```python
from build123d import *

# Parameters (mm, degrees)
F1_DEPTH       = 12.065
F2_R           = 9.525
F3_DEPTH       = 15.25
F4_R           = 9.625
F5_DEPTH       = 25
F7_D           = 9
F7_DEPTH       = 75
F7_CBORE_D     = 11
F7_CBORE_DEPTH = 5
F7_TIP         = 2.7038727856
F8_R           = 2.5


# Not quite as in the source:
# - a pattern or mirror of a feature is missing from the dataset's text; its kind, count and spacing are read off the source's solid


with BuildPart() as f1:
    # F0 (on Right) → F1 (new body, symmetric)
    with BuildSketch(Plane.YZ):
        with BuildLine():
            ThreePointArc((-38.1, 0), (0, 38.1), (38.1, 0))
            Line((38.1, 0), (50.8, 0))
            ThreePointArc((50.8, 0), (0, 50.8), (-50.8, 0))
            Line((-50.8, 0), (-38.1, 0))
        make_face()
    extrude(amount=F1_DEPTH, both=True)

    # F2 (on face) → F3 (join)
    with BuildSketch(Plane(origin=(0, 0, 0), x_dir=(1, 0, 0), z_dir=(0, 0, -1))):
        with Locations((0, -50.8)):
            Circle(F2_R)
    f3 = extrude(amount=-F3_DEPTH)

    # F3_copies: F3 across plane
    add(f3.mirror(Plane(origin=(0, 0, 0), x_dir=(0, 0, -1), z_dir=(0, -1, 0))))

    # F4 (on face) → F5 (cut)
    with BuildSketch(Plane.XY.offset(15.25)):
        with Locations((0, 50.8)):
            Circle(F4_R)
    f5 = extrude(amount=F5_DEPTH, mode=Mode.SUBTRACT)

    # F5_copies: F5 across plane
    add(f5.mirror(Plane(origin=(0, -4e-06, 0), x_dir=(0, 0, -1), z_dir=(0, -1, 0))), mode=Mode.SUBTRACT)

    # F7
    with Locations(Plane.XY.offset(15.25)):
        with Locations((0, 50.8)):
            f7 = CounterBoreHole(F7_D / 2, F7_CBORE_D / 2, F7_CBORE_DEPTH, depth=F7_DEPTH)
            with Locations((0, 0, -(F7_DEPTH + F7_TIP / 2))):  # 118° drill point
                Cone(0, F7_D / 2, F7_TIP, mode=Mode.SUBTRACT)

    # F7_copies: F7 across plane
    add(f7.mirror(Plane(origin=(0, 0, 0), x_dir=(0, 0, -1), z_dir=(0, -1, 0))), mode=Mode.SUBTRACT)

    # F8
    f8_edges = [f1.edges().sort_by_distance(p)[0] for p in [
        (12.065, 0, 50.8),
        (-12.065, 0, 50.8),
    ]]
    fillet(f8_edges, radius=F8_R)


solid = f1.part
```
The model under review builds one solid part; all positions refer to its coordinate system, in mm. A direction names the side the tool comes from. Give positions to 0.01 mm unless a question says otherwise; leave off trailing zeros. Loops run counter-clockwise (first coordinate to the right, second up) from the corner with the lowest first, then second, coordinate; pieces in that order, holes last. Notation, with made-up numbers: (65.25, -12.5) -> (88.25, -12.5) arc R20 ccw to (88.25, -6.5) -> close; hole circle Ø5 at (-20, 86). An arc over 180 degrees is marked (long way). Use CSV: the item, a comma, the result in double quotes.
1. To check wall thickness, follow probe 1 along X at (y, z) = (-50.8, 5) (3 decimals); probe 2 along Y at (x, z) = (0, 6.25) (3 decimals); probe 3 along Y at (x, z) = (0, 5.5) (3 decimals). State the ranges of each line that lie inside material, in increasing order. Write a range as from..to.
Result:
probe 1,"x = -9.525..-4.5, 4.5..9.525"
probe 2,"y = -60.325..-55.3, -46.3..-37.584, 37.584..46.3, 55.3..60.325"
probe 3,"y = -60.325..-55.3, -46.3..-37.701, 37.701..46.3, 55.3..60.325"
2. Consider section A-A, the plane x = 0. Write out the cut boundary in (y, z) (3 decimals).
Result:
outline,"(-60.325, 0) -> (-55.3, 0) -> (-55.3, 10.25) -> (-56.3, 10.25) -> (-56.3, 15.25) -> (-60.325, 15.25) -> close; (-46.3, 0) -> (-38.1, 0) arc R38.1 cw to (38.1, 0) -> (46.3, 0) -> (46.3, 10.25) -> (45.3, 10.25) -> (45.3, 15.25) -> (41.175, 15.25) -> (41.175, 29.753) arc R50.8 ccw to (-41.175, 29.753) -> (-41.175, 15.25) -> (-45.3, 15.25) -> (-45.3, 10.25) -> (-46.3, 10.25) -> close; (55.3, 0) -> (60.325, 0) -> (60.325, 15.25) -> (56.3, 15.25) -> (56.3, 10.25) -> (55.3, 10.25) -> close"
3. Consider section B-B, the plane y = 0. Write out the cut boundary in (x, z) (3 decimals).
Result:
outline,"(-12.065, 38.1) -> (12.065, 38.1) -> (12.065, 48.3) arc R2.5 ccw to (9.565, 50.8) -> (-9.565, 50.8) arc R2.5 ccw to (-12.065, 48.3) -> close"
4. The part is to be moulded in two halves that separate along Y. For faces 6 (the face through (4.1, 46.6, 15.25)), 7 (the face through (-0.179, -41.177, 20.789)), 8 (the face through (-5, -51, 10.25)), say which applies: +Y half, -Y half, draft (parallel to the pull), parting line (faces both ways), or undercut.
Result:
face 6,"draft"
face 7,"-Y half"
face 8,"undercut"
5. For P1, Ø6, axis at x = -1, y = -19, coming from the +Z side; P2, Ø1, axis at x = -9, z = 20, coming from the -Y side; P3, Ø10.5, axis at x = 0, y = -50.8, coming from the +Z side, all flat-tipped, find the tip position at first contact; note any pin that passes through.
Result:
P1,"stops at z = 48.21"
P2,"stops at y = -46.91"
P3,"stops at z = 10.25"
6. Machinability: for faces 1 (the face through (4, -55, 15.25)), 2 (the face through (-0.716, -56.253, 12.785)), 3 (the face through (3, 47, 0)), 4 (the face through (-12.065, 3, 39)), 5 (the face through (-0.179, 41.177, 20.789)), which of the approach directions +Z, -Z, +X, -X, +Y, -Y give a long, thin tool a straight path to every point of the face, cutting with its end or side? Answer none if there is none.
Result:
face 1,"+Z, -Y"
face 2,"+Z"
face 3,"-Z, +X, -X, +Y, -Y"
face 4,"+Z, -Z, -X, +Y, -Y"
face 5,"+Z, +Y"
